from build123d import *

# Parameters (mm, degrees)
BOSS_EXTRUDE1_DEPTH = 0.85
FILLET1_R           = 1


with BuildPart() as part:
    # Sketch1 → Boss-Extrude1 (new, symmetric)
    with BuildSketch(Plane(origin=(0, 0, 0), x_dir=(1, 0, 0), z_dir=(0, 1, 0))):
        with BuildLine():
            Line((-10.133853114, -10.590839948), (-19.119202876, -0.785051368))
            ThreePointArc((-19.119202876, -0.785051368), (0, 6.65), (19.119202876, -0.785051368))
            Line((19.119202876, -0.785051368), (10.133853114, -10.590839948))
            ThreePointArc((10.133853114, -10.590839948), (0, -6.65), (-10.133853114, -10.590839948))
        make_face()
    extrude(amount=BOSS_EXTRUDE1_DEPTH, both=True)

    # Fillet1
    fillet1_edges = [part.edges().sort_by_distance(p)[0] for p in [
        (-10.133853114, 0, 10.590839948),
        (-19.119202876, 0, 0.785051368),
        (19.119202876, 0, 0.785051368),
        (10.133853114, 0, 10.590839948),
    ]]
    fillet(fillet1_edges, radius=FILLET1_R)


solid = part.part
Input: part model. Units: mm. Frame: model coordinates. Give positions to 0.01 mm unless a question says otherwise; leave off trailing zeros. Loops run counter-clockwise (first coordinate to the right, second up) from the corner with the lowest first, then second, coordinate; pieces in that order, holes last. Notation, with made-up numbers: M 37,17.5 L 46,17.5 A26 cw 46,43.5 Z; hole C 87.5,78 d1. An arc over 180 degrees is marked long. Use one line per item in the form item = value.
1. Line query: L1, parallel to Z at x = 0.5, y = -0.5; L2, parallel to X at y = 0.25, z = 9.25; L3, parallel to X at y = 0.7, z = -0.5. Output: solid intervals per line, ascending.
Numbers:
L1 = -6.65 to 6.66
L2 = -11.36 to -8.44, 8.44 to 11.36
L3 = -17.61 to 17.61
2. Section query D-D, the plane z = -5. Return the cut outline in (x, y), and give its area (3 significant figures).
Numbers:
outline = M -9.52,-0.85 L 9.52,-0.85 L 9.52,0.85 L -9.52,0.85 Z
area = 32.4 mm²
3. Section query B-B, the plane z = 8.5. Return the cut outline in (x, y).
Numbers:
outline = M -12.05,-0.85 L -7.22,-0.85 L -7.22,0.85 L -12.05,0.85 Z; M 7.22,-0.85 L 12.05,-0.85 L 12.05,0.85 L 7.22,0.85 Z
4. First-contact query: pin 1 (1 mm diameter, centred on y = 0.5, z = -4, fed in from -X). Flat tip, straight axial feed; report the tip coordinate or a pass-through.
Numbers:
pin_1 = -12.98
5. Section query A-A, the plane y = 0.35. Return the cut outline in (x, z).
Numbers:
outline = M -18.43,1.54 A1 ccw -18.34,0.1 A28.3 ccw 18.34,0.1 A1 ccw 18.43,1.54 L 10.79,9.88 A1 ccw 9.42,9.98 A15 cw -9.42,9.98 A1 ccw -10.79,9.88 Z
6. Pull-direction query (X, two-part tool) for faces 1 (the face through (0, -0.85, 2)), 2 (the face through (18.693, -0.012, 0.81)), 3 (the face through (0.14, 0.01, 6.65)); classes: released by +X, released by -X, zero draft, split by the parting line, or undercut.
Numbers:
face_1 = zero draft
face_2 = released by +X
face_3 = undercut
7. Section query C-C, the plane x = 13. Return the cut outline in (y, z).
Numbers:
outline = M -0.85,-3.49 L 0.85,-3.49 L 0.85,7.46 L -0.85,7.46 Z
